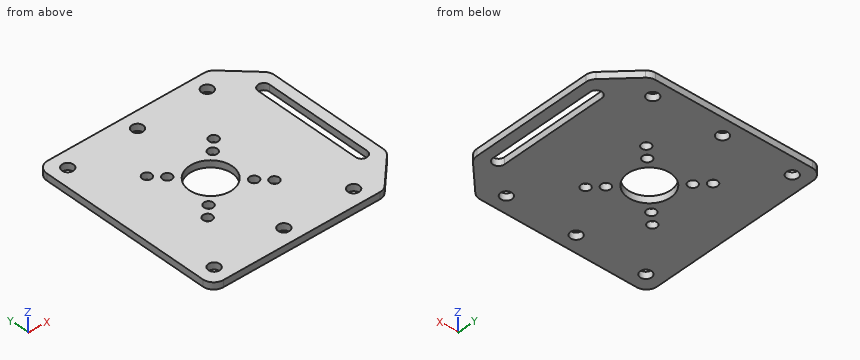
from build123d import *

# Parameters (mm, degrees)
SKETCH1_R            = 10
BASE_FLANGE1_DEPTH   = 3.175
M4_CLEARANCE_HOLE1_D = 4.3
M5_CLEARANCE_HOLE1_D = 5.3
FILLET1_R            = 5


# Sheet-metal steps are written as plain solids
with BuildPart() as part:
    # Sketch1 → Base-Flange1 (new body)
    with BuildSketch(Plane.XY):
        Polygon((40, 45), (55, 30), (55, -30), (40, -45), (-40, -45), (-40, 45), align=None)
        Circle(SKETCH1_R, mode=Mode.SUBTRACT)
        with BuildLine():
            Line((44.85, 25), (44.85, -25))
            ThreePointArc((44.85, -25), (47.5, -27.65), (50.15, -25))
            Line((50.15, -25), (50.15, 25))
            ThreePointArc((50.15, 25), (47.5, 27.65), (44.85, 25))
        make_face(mode=Mode.SUBTRACT)
    extrude(amount=-BASE_FLANGE1_DEPTH)

    # M4 Clearance Hole1 (through all)
    with Locations(Plane(origin=(-15.556349186, 15.556349186, 0), x_dir=(1, 0, 0), z_dir=(0, 0, 1))):
        with Locations((0, 0), (31.112698372, 0), (26.162950904, -4.949747468), (4.949747468, -4.949747468), (0, -31.112698372), (31.112698372, -31.112698372), (26.162950904, -26.162950904), (4.949747468, -26.162950904)):
            Hole(M4_CLEARANCE_HOLE1_D / 2)

    # M5 Clearance Hole1 (through all)
    with Locations(Plane(origin=(-32.5, 37.5, 0), x_dir=(1, 0, 0), z_dir=(0, 0, 1))):
        with Locations((0, 0), (65, 0), (65, -75), (0, -75), (32.5, 0), (32.5, -75)):
            Hole(M5_CLEARANCE_HOLE1_D / 2)

    # Fillet1
    fillet1_edges = [part.edges().sort_by_distance(p)[0] for p in [
        (-40, 45, -1.5875),
        (40, 45, -1.5875),
        (55, 30, -1.5875),
        (55, -30, -1.5875),
        (40, -45, -1.5875),
        (-40, -45, -1.5875),
    ]]
    fillet(fillet1_edges, radius=FILLET1_R)


solid = part.part
Design review of the part built by this model. Coordinates are the model's own, in mm. Round coordinates to 2 decimals unless told otherwise and drop trailing zeros. Write each loop counter-clockwise with the first axis right and the second up, starting at its lowest first coordinate (ties: lowest second). Pieces come first, ordered by that corner, then holes. Notation, with made-up numbers: (85.25, 75) - (129.25, 75) arc R28 cw to (129.25, 97) - close; hole circle Ø4 at (40.25, -18). An arc over 180 degrees is marked (long way). Use a Markdown table: item, result. Add a question column.
1. We need section C-C (y = -37.5). State the section outline as (x, z) points (3 decimals).
2. We need section A-A (x = -32.5). State the section outline as (y, z) points (3 decimals), then the cut area to 3 significant figures.
3. We need section B-B (x = -6). State the section outline as (y, z) points (3 decimals), then the cut area to 3 significant figures.
4. We need section D-D (y = 0). State the section outline as (x, z) points (3 decimals), then the cut area to 3 significant figures.
5. Wall thickness on probe 1 along X at (y, z) = (-0.5, -0.7); probe 2 along X at (y, z) = (-18, -2.55); probe 3 along X at (y, z) = (39, -2.6): over which ranges is each line inside the solid? List them lowest first.
Output:
| question | item | result |
|---|---|---|
| 1 | outline | (-40, -3.175) - (-35.15, -3.175) - (-35.15, 0) - (-40, 0) - close; (-29.85, -3.175) - (-2.65, -3.175) - (-2.65, 0) - (-29.85, 0) - close; (2.65, -3.175) - (29.85, -3.175) - (29.85, 0) - (2.65, 0) - close; (35.15, -3.175) - (47.5, -3.175) - (47.5, 0) - (35.15, 0) - close |
| 2 | outline | (-45, -3.175) - (-40.15, -3.175) - (-40.15, 0) - (-45, 0) - close; (-34.85, -3.175) - (34.85, -3.175) - (34.85, 0) - (-34.85, 0) - close; (40.15, -3.175) - (45, -3.175) - (45, 0) - (40.15, 0) - close |
| 2 | area | 252 mm2 |
| 3 | outline | (-45, -3.175) - (-8, -3.175) - (-8, 0) - (-45, 0) - close; (8, -3.175) - (45, -3.175) - (45, 0) - (8, 0) - close |
| 3 | area | 235 mm2 |
| 4 | outline | (-40, -3.175) - (-10, -3.175) - (-10, 0) - (-40, 0) - close; (10, -3.175) - (44.85, -3.175) - (44.85, 0) - (10, 0) - close; (50.15, -3.175) - (55, -3.175) - (55, 0) - (50.15, 0) - close |
| 4 | area | 221 mm2 |
| 5 | probe 1 | x = -40 to -9.99, 9.99 to 44.85, 50.15 to 55 |
| 5 | probe 2 | x = -40 to 44.85, 50.15 to 55 |
| 5 | probe 3 | x = -40 to -34.68, -30.32 to -2.18, 2.18 to 30.32, 34.68 to 46 |
